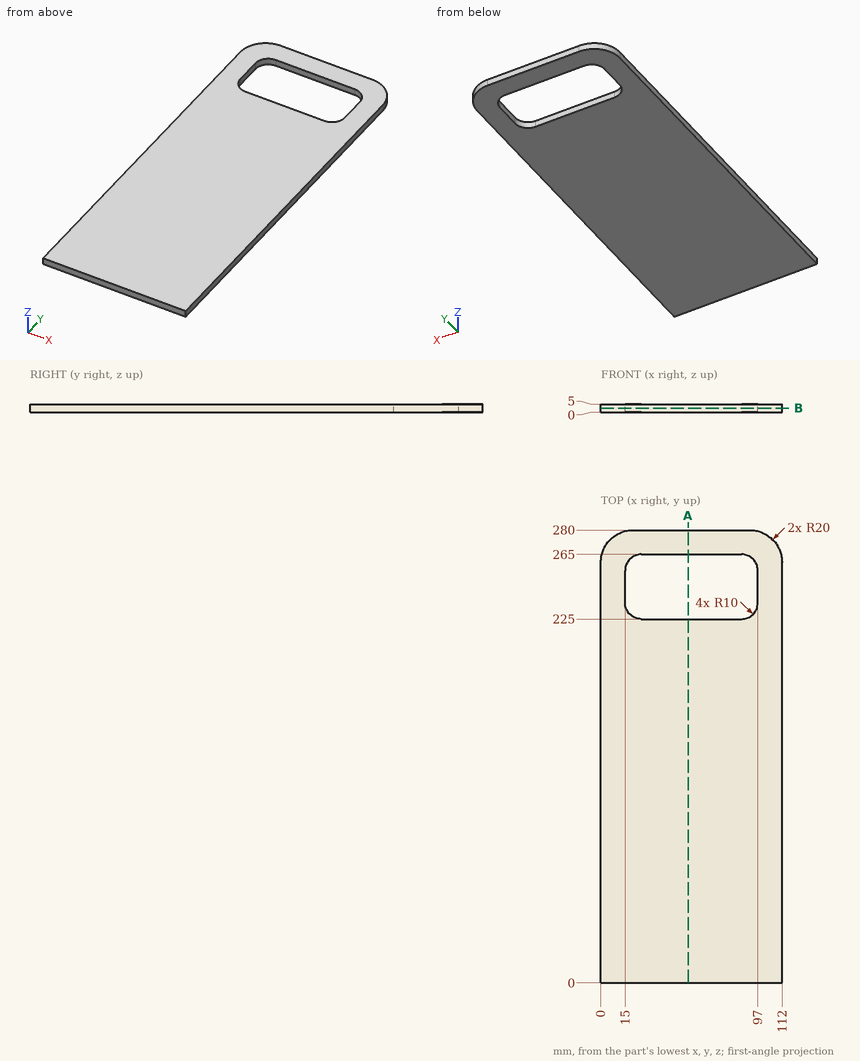
Answer from the drawing. Dimensions are ordinates in mm from the lowest x, y and z of the part. Coordinates: 2 decimals unless noted, no trailing zeros. Loops run counter-clockwise (first coordinate to the right, second up) from the corner with the lowest first, then second, coordinate; pieces in that order, holes last. Notation, with made-up numbers: (-10, 27) - (36, 27) arc R23 ccw to (36, 45) - close; hole circle Ø11 at (8.25, -27). An arc over 180 degrees is marked (long way). Answer in a Markdown table with one row per item.
1. Find section B-B, the plane z = 2.5. Write down the section's boundary in (x, y), then the cut area to 3 significant figures.
Conclusion:
| item | result |
|---|---|
| outline | (0, 0) - (112, 0) - (112, 260) arc R20 ccw to (92, 280) - (20, 280) arc R20 ccw to (0, 260) - close; hole (15, 235) arc R10 ccw to (25, 225) - (87, 225) arc R10 ccw to (97, 235) - (97, 255) arc R10 ccw to (87, 265) - (25, 265) arc R10 ccw to (15, 255) - close |
| area | 28,000 mm² |
2. Straight lines are drawn through the part: line 1 (Y direction, x = 86.5, z = 0.7); line 2 (X direction, y = 233.5, z = 2.1); line 3 (Y direction, x = 22, z = 3.9). For each, find the intervals that lie inside material, in ascending order.
Conclusion:
| item | result |
|---|---|
| line 1 | y = 0 to 225, 265 to 280 |
| line 2 | x = 0 to 15.11, 96.89 to 112 |
| line 3 | y = 0 to 225.46, 264.54 to 280 |
3. Find section A-A, the plane x = 54. Write down the section's boundary in (y, z).
Conclusion:
| item | result |
|---|---|
| outline | (0, 0) - (225, 0) - (225, 5) - (0, 5) - close; (265, 0) - (280, 0) - (280, 5) - (265, 5) - close |
